```python
from build123d import *

# Parameters (mm, degrees)
SKETCH1_W                                        = 45
SKETCH1_H                                        = 45
BASE_DEPTH                                       = 6
CBORE_FOR_M4_HEX_HEAD_MACHINE_SCREW1_D           = 4.5
CBORE_FOR_M4_HEX_HEAD_MACHINE_SCREW1_CBORE_D     = 10.59
CBORE_FOR_M4_HEX_HEAD_MACHINE_SCREW1_CBORE_DEPTH = 3
SKETCH4_W                                        = 35
SKETCH4_H                                        = 6
STANDING_PLATFORM_DEPTH                          = 25
FRONT_ARM_DEPTH                                  = 7.5
SKETCH6_R                                        = 3
STEERING_HOLE_DEPTH                              = 15
FILLET1_R                                        = 6


with BuildPart() as part:
    # Sketch1 → BASE (new body)
    with BuildSketch(Plane(origin=(0, 0, 0), x_dir=(1, 0, 0), z_dir=(0, 1, 0))):
        Rectangle(SKETCH1_W, SKETCH1_H)
    extrude(amount=-BASE_DEPTH)

    # CBORE for M4 Hex Head Machine Screw1 (through all)
    with Locations(Plane(origin=(0, -6, 0), x_dir=(-1, 0, 0), z_dir=(0, -1, 0))):
        with Locations((10, -10), (-10, -10), (-10, 10), (10, 10)):
            CounterBoreHole(CBORE_FOR_M4_HEX_HEAD_MACHINE_SCREW1_D / 2, CBORE_FOR_M4_HEX_HEAD_MACHINE_SCREW1_CBORE_D / 2, CBORE_FOR_M4_HEX_HEAD_MACHINE_SCREW1_CBORE_DEPTH)

    # Sketch4 → Standing Platform (add)
    with BuildSketch(Plane(origin=(22.5, 0, 0), x_dir=(0, 0, -1), z_dir=(1, 0, 0))):
        with Locations((0, -3)):
            Rectangle(SKETCH4_W, SKETCH4_H)
    extrude(amount=STANDING_PLATFORM_DEPTH)

    # Sketch5 → Front Arm (add, symmetric)
    with BuildSketch(Plane.XY):
        Polygon((47.5, -6), (67.5, 54), (102.5, 54), (102.5, 60), (63.17544468, 60), (41.17544468, -6), align=None)
    extrude(amount=FRONT_ARM_DEPTH, both=True)

    # Sketch6 → Steering Hole (cut)
    with BuildSketch(Plane(origin=(0, 60, 0), x_dir=(1, 0, 0), z_dir=(0, 1, 0))):
        with Locations(Location((93.5, 0, 0), (0, 0, 270))):
            Circle(SKETCH6_R)
    extrude(amount=-STEERING_HOLE_DEPTH, mode=Mode.SUBTRACT)

    # Fillet1
    fillet1_edges = [part.edges().sort_by_distance(p)[0] for p in [
        (102.5, 57, 7.5),
        (102.5, 57, -7.5),
    ]]
    fillet(fillet1_edges, radius=FILLET1_R)


solid = part.part
```
Check sheet for the modelled part. Datum: model origin and axes. Units: mm. A direction names the side the tool comes from. Round coordinates to 2 decimals unless told otherwise and drop trailing zeros. Loops run counter-clockwise (first coordinate to the right, second up) from the corner with the lowest first, then second, coordinate; pieces in that order, holes last. Notation, with made-up numbers: (-32, -8) -> (-11, -8) arc R32 ccw to (-11, 30) -> close; hole circle Ø11 at (16.5, -4). An arc over 180 degrees is marked (long way). Write item = value, one per line. Start each with the question number.
1) Set-up check for faces 4 (the flat face through (53.315, 30.42, 0.105)), 5 (the flat face through (85, 54, 0)), 6 (the flat face through (22.5, -3, -20)), 7 (the flat face through (35, -3, 17.5)), 8 (the cylindrical face through (-12.44, -4.52, -5.3)): record each of +Z, -Z, +X, -X, +Y, -Y from which the full face is reachable in a straight line by a thin tool's end or side.
2) Sectioned sample at D-D, the plane x = -10. Record the cut outline in (y, z) (3 decimals).
3) Sectioned sample at C-C, the plane z = -10. Record the cut outline in (x, y) (3 decimals), plus the area to 3 significant figures.
4) Thickness scan on probe 1 along X at (y, z) = (-2, -10); probe 2 along Z at (x, y) = (10, -4.7) (3 decimals); probe 3 along X at (y, z) = (-2.5, -11). Record the ranges inside material, lowest first.
5) Gauge pin test, flat ends, axial feed: pin 1 Ø5 at (x, z) = (-10, 10) entering from +Y; pin 2 Ø4 at (y, z) = (29.5, -6.5) entering from +X; pin 3 Ø6.5 at (x, y) = (40.5, -3.5) entering from +Z. Record the tip position at first contact, or that the pin passes through.
6) Sectioned sample at B-B, the plane x = 93.5. Record the cut outline in (y, z), plus the area to 3 significant figures.
7) Sectioned sample at A-A, the plane z = 0. Record the cut outline in (x, y), plus the area to 3 significant figures.
8) Release check for a two-part mould opening along Z. For faces 1 (the flat face through (-11.1, -3, 12.3)), 2 (the flat face through (0, -3, 22.5)), 3 (the flat face through (102.5, 57, 0)) record: released by +Z, released by -Z, zero draft, split by the parting line, or undercut.
Results are:
q1.face_4 = +Z, -Z, -X, +Y
q1.face_5 = +Z, -Z, +X, -Y
q1.face_6 = -Z, +X, +Y, -Y
q1.face_7 = +Z, +X, +Y, -Y
q1.face_8 = -Y
q2.outline = (-6, -22.5) -> (0, -22.5) -> (0, -12.25) -> (-3, -12.25) -> (-3, -15.295) -> (-6, -15.295) -> close; (-6, -4.705) -> (-3, -4.705) -> (-3, -7.75) -> (0, -7.75) -> (0, 7.75) -> (-3, 7.75) -> (-3, 4.705) -> (-6, 4.705) -> close; (-6, 15.295) -> (-3, 15.295) -> (-3, 12.25) -> (0, 12.25) -> (0, 22.5) -> (-6, 22.5) -> close
q3.outline = (-22.5, -6) -> (-15.295, -6) -> (-15.295, -3) -> (-12.25, -3) -> (-12.25, 0) -> (-22.5, 0) -> close; (-7.75, -3) -> (-4.705, -3) -> (-4.705, -6) -> (4.705, -6) -> (4.705, -3) -> (7.75, -3) -> (7.75, 0) -> (-7.75, 0) -> close; (12.25, -3) -> (15.295, -3) -> (15.295, -6) -> (47.5, -6) -> (47.5, 0) -> (12.25, 0) -> close
q3.area = 329 mm^2
q4.probe_1 = -22.5 to -12.25, -7.75 to 7.75, 12.25 to 47.5
q4.probe_2 = -22.5 to -15.295, -4.705 to 4.705, 15.295 to 22.5
q4.probe_3 = -22.5 to -12.02, -7.98 to 7.98, 12.02 to 47.5
q5.pin_1 = 0
q5.pin_2 = 60
q5.pin_3 = 17.5
q6.outline = (54, -7.5) -> (60, -7.5) -> (60, -3) -> (54, -3) -> close; (54, 3) -> (60, 3) -> (60, 7.5) -> (54, 7.5) -> close
q6.area = 54.0 mm^2
q7.outline = (-22.5, -6) -> (47.5, -6) -> (67.5, 54) -> (90.5, 54) -> (90.5, 60) -> (63.18, 60) -> (43.18, 0) -> (-22.5, 0) -> close; (96.5, 54) -> (102.5, 54) -> (102.5, 60) -> (96.5, 60) -> close
q7.area = 973 mm^2
q8.face_1 = undercut
q8.face_2 = released by +Z
q8.face_3 = zero draft
